The drawing under review shows one solid part. Ordinate dimensions are in mm from its lowest x, y, z. A direction names the side the tool comes from. Round coordinates to 2 decimals unless told otherwise and drop trailing zeros. Order: outer loops, then holes, each group sorted by start corner. A loop starts at its lowest first (then second) coordinate and runs counter-clockwise, first axis right, second up. Notation, with made-up numbers: (-37.75, -22) -> (-18.75, -22) arc R13 ccw to (-18.75, -12) -> close; hole circle Ø4 at (-17, -40). An arc over 180 degrees is marked (long way). Use a Markdown table: item, result. Add a question column.
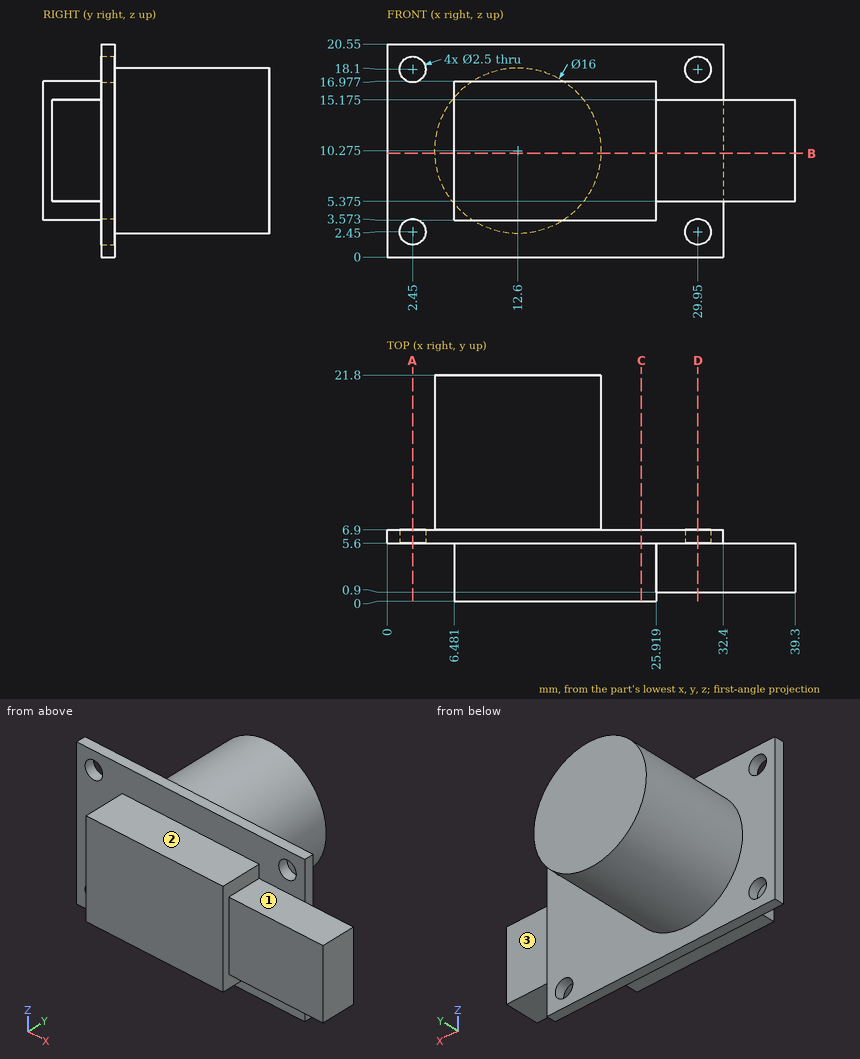
Q1. For the marked faces 1, 2 and 3, list the 3-axis set-ups (+Z, -Z, +X, -X, +Y, -Y) from which the entire face can be reached by the end or side of a thin tool; tool diameter is ignored.
Q2. Add section A-A, the plane x = 2.45. Give the boundary of the cut face in (y, z).
Q3. For pin 1 (6 mm diameter, centred on y = 2, z = 10, fed in from -X); pin 2 (6 mm diameter, centred on x = 23, y = 18, fed in from +Z) (1 decimal); pin 3 (3 mm diameter, centred on x = 34.5, z = 10, fed in from -Y), all flat-tipped, find the tip position at first contact; note any pin that passes through.
Q4. Add section D-D, the plane x = 29.95. Give the number of separate pieces and of enclosed holes in the cut face.
Q5. Add section C-C, the plane x = 24.5. Give the boundary of the cut face in (y, z), then the cut area to 3 significant figures.
Q6. To check wall thickness, follow line 1 along X through (y, z) = (6.6, 2.45); line 2 along Y through (x, z) = (21.5, 3.5); line 3 along X through (y, z) = (4.5, 11.5). State the ranges of each line that lie inside material, in increasing order.
Q7. Add section B-B, the plane z = 10. Give the boundary of the cut face in (x, y) (1 decimal).
Return value:
| question | item | result |
|---|---|---|
| 1 | face 1 | +Z, +X, -Y |
| 1 | face 2 | +Z, +X, -X, -Y |
| 1 | face 3 | +Z, -Z, +X, +Y |
| 2 | outline | (5.6, 0) -> (6.9, 0) -> (6.9, 1.2) -> (5.6, 1.2) -> close; (5.6, 3.7) -> (6.9, 3.7) -> (6.9, 16.85) -> (5.6, 16.85) -> close; (5.6, 19.35) -> (6.9, 19.35) -> (6.9, 20.55) -> (5.6, 20.55) -> close |
| 3 | pin 1 | x = 6.48 |
| 3 | pin 2 | z = 13.3 |
| 3 | pin 3 | y = 0.9 |
| 4 | separate pieces | 3 |
| 4 | enclosed holes | 0 |
| 5 | outline | (0, 3.57) -> (5.6, 3.57) -> (5.6, 0) -> (6.9, 0) -> (6.9, 20.55) -> (5.6, 20.55) -> (5.6, 16.98) -> (0, 16.98) -> close |
| 5 | area | 102 mm² |
| 6 | line 1 | 0 to 1.2, 3.7 to 28.7, 31.2 to 32.4 |
| 6 | line 2 | 5.6 to 6.9 |
| 6 | line 3 | 6.48 to 39.3 |
| 7 | outline | (0, 5.6) -> (6.5, 5.6) -> (6.5, 0) -> (25.9, 0) -> (25.9, 0.9) -> (39.3, 0.9) -> (39.3, 5.6) -> (32.4, 5.6) -> (32.4, 6.9) -> (20.6, 6.9) -> (20.6, 21.8) -> (4.6, 21.8) -> (4.6, 6.9) -> (0, 6.9) -> close |
